Geometry: see drawing. Coordinates: mm, zero at the bounding-box minimum. A direction names the side the tool comes from. Coordinates: 2 decimals unless noted, no trailing zeros. Write each loop counter-clockwise with the first axis right and the second up, starting at its lowest first coordinate (ties: lowest second). Pieces come first, ordered by that corner, then holes. Notation, with made-up numbers: (-19.5, 38.25) - (28.5, 38.25) arc R17 cw to (28.5, 60.25) - close; hole circle Ø4 at (-35.75, 71). An arc over 180 degrees is marked (long way). Use CSV: the item, a comma, the result in double quotes.
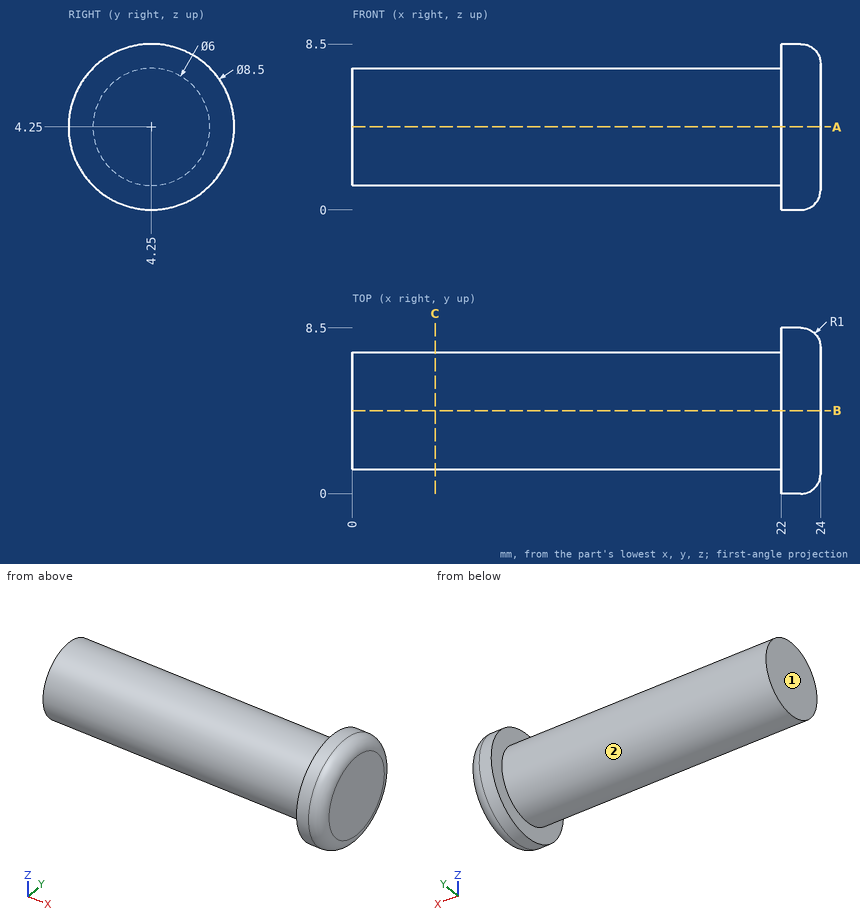
(1) Cut plane C-C on x = 4.25. Return loops of the section in (y, z), and give its area (3 significant figures).
Check values:
outline,"circle Ø6 at (4.25, 4.25)"
area,"28.3 mm^2"
(2) Ray query, probe 1 along X at (y, z) = (1.25, 5); probe 2 along Y at (x, z) = (21.5, 6.25); probe 3 along Y at (x, z) = (16.75, 3.75). Return the intervals inside material, ascending. Write a range as from..to.
Check values:
probe 1,"22..24"
probe 2,"2.01..6.49"
probe 3,"1.29..7.21"
(3) Reachability of the marked faces 1 and 2 from +Z, -Z, +X, -X, +Y, -Y: full face, straight path, thin tool, end or side. Return the list, or none.
Check values:
face 1,"+Z, -Z, -X, +Y, -Y"
face 2,"-X"
(4) Cut plane A-A on z = 4.25. Return loops of the section in (x, y), and give its area (3 significant figures).
Check values:
outline,"(0, 1.25) - (22, 1.25) - (22, 0) - (23, 0) arc R1 ccw to (24, 1) - (24, 7.5) arc R1 ccw to (23, 8.5) - (22, 8.5) - (22, 7.25) - (0, 7.25) - close"
area,"149 mm^2"
(5) Pin query (flat end, axial travel): pin 1 Ø5 at (x, y) = (5, 5.5) entering from +Z. Return the tip coordinate at first contact, or that it passes through.
Check values:
pin 1,"z = 7.25"
